Read the model definition and answer for the solid it produces. Units are mm, in the model's axes. Face numbers are marked on the shaded views. A direction names the side the tool comes from. Coordinates: 2 decimals unless noted, no trailing zeros. Order: outer loops, then holes, each group sorted by start corner. A loop starts at its lowest first (then second) coordinate and runs counter-clockwise, first axis right, second up. Notation, with made-up numbers: (-1.5, -17.5) -> (35.5, -17.5) arc R30 cw to (35.5, 17.5) -> close; hole circle Ø4 at (-36, 13). An arc over 180 degrees is marked (long way). Use CSV: the item, a comma, the result in double quotes.
```python
from build123d import *

# Parameters (mm, degrees)
EXTRUDE_1_DEPTH     = 14
SKETCH_3_W          = 34.989164417
SKETCH_3_H          = 23.7
EXTRUDE_2_DEPTH     = 1.99
SKETCH_4_W          = 19.73952378
SKETCH_4_H          = 14
CUT_EXTRUDE_1_DEPTH = 1.99
EXTRUDE_3_DEPTH     = 4.99
EXTRUDE_4_DEPTH     = 5.55
EXTRUDE_5_DEPTH     = 1.02
SKETCH_13_W         = 35
SKETCH_13_H         = 14
EXTRUDE_6_DEPTH     = 4
EXTRUDE_8_DEPTH     = 21
SKETCH_15_W         = 5
SKETCH_15_H         = 5.74
SKETCH_15_H_2       = 4
EXTRUDE_9_DEPTH     = 14
EXTRUDE_10_DEPTH    = 1
SKETCH_17_W         = 35
SKETCH_17_H         = 19
EXTRUDE_11_DEPTH    = 3
SKETCH_18_W         = 35
SKETCH_18_H         = 5
EXTRUDE_12_DEPTH    = 1
EXTRUDE_16_DEPTH    = 3
SKETCH_20_W         = 5.25
SKETCH_20_H         = 3.26
SKETCH_20_H_2       = 3
EXTRUDE_18_DEPTH    = 35
SKETCH_21_W         = 14
SKETCH_21_H         = 3.74
SKETCH_21_H_2       = 3.75
EXTRUDE_19_DEPTH    = 5
EXTRUDE_20_DEPTH    = 11
SKETCH_26_W         = 0.25
SKETCH_26_H         = 8.5
EXTRUDE_21_DEPTH    = 3
SKETCH_27_W         = 21
SKETCH_27_H         = 8.5
EXTRUDE_22_DEPTH    = 80
SKETCH_28_R         = 25
SKETCH_28_R_2       = 6
SKETCH_28_R_3       = 1.5
EXTRUDE_23_DEPTH    = 3


with BuildPart() as part:
    # 草图2 → 凸台-拉伸1 (new body)
    with BuildSketch(Plane.XY.offset(6)):
        Polygon((58.617261146, 15.562420382), (53.219585402, 15.562420382), (53.219585402, 12.262420382), (57.419585402, 12.262420382), (57.419585402, 8.862420382), (53.219585402, 8.862420382), (53.219585402, -6.137579618), (29.014936891, -6.137579618), (29.014936891, 8.862420382), (24.814936891, 8.862420382), (24.814936891, 12.262420382), (29.014936891, 12.262420382), (29.014936891, 15.562420382), (23.617261146, 15.562420382), (23.617261146, -8.137579618), (58.617261146, -8.137579618), align=None)
    extrude(amount=-EXTRUDE_1_DEPTH)

    # 草图3 → 凸台-拉伸2 (add)
    with BuildSketch(Plane(origin=(0, 0, -8), x_dir=(-1, 0, 0), z_dir=(0, 0, -1))):
        with Locations((-41.122678938, 3.712420382)):
            Rectangle(SKETCH_3_W, SKETCH_3_H)
    extrude(amount=-EXTRUDE_2_DEPTH)

    # 草图4 → 切除-拉伸1 (cut)
    with BuildSketch(Plane.XZ.offset(8.137579618)):
        with Locations((41.002259963, -1)):
            Rectangle(SKETCH_4_W, SKETCH_4_H)
    extrude(amount=-CUT_EXTRUDE_1_DEPTH, mode=Mode.SUBTRACT)

    # 草图7 → 凸台-拉伸3 (add)
    with BuildSketch(Plane(origin=(0, 15.562420382, 0), x_dir=(1, 0, 0), z_dir=(0, 1, 0))):
        Polygon((29.014936891, -6), (23.617261146, -6), (23.617261146, 8), (58.617261146, 8), (58.617261146, -6), (53.219585402, -6), (53.219585402, 6.01), (29.014936891, 6.01), align=None)
    extrude(amount=EXTRUDE_3_DEPTH)

    # 草图8 → 凸台-拉伸4 (add)
    with BuildSketch(Plane(origin=(0, 20.552420382, 0), x_dir=(1, 0, 0), z_dir=(0, 1, 0))):
        Polygon((23.617261146, -6), (29.014936891, -6), (29.014936891, 6.01), (44.953536614, 6.01), (44.953536614, -6), (58.617261146, -6), (58.617261146, 8), (23.617261146, 8), align=None)
    extrude(amount=EXTRUDE_4_DEPTH)

    # 草图11 → 凸台-拉伸5 (add)
    with BuildSketch(Plane(origin=(0, 26.102420382, 0), x_dir=(1, 0, 0), z_dir=(0, 1, 0))):
        with BuildLine():
            Line((51.35010895, 8), (58.617261146, 8))
            Line((58.617261146, 8), (58.617261146, -6))
            Line((58.617261146, -6), (52.21613159, -6))
            ThreePointArc((52.21613159, -6), (53.233588834, 1.089724187), (51.35010895, 8))
        make_face()
    extrude(amount=EXTRUDE_5_DEPTH)

    # 草图13 → 凸台-拉伸6 (add)
    with BuildSketch(Plane(origin=(0, 27.122420382, 0), x_dir=(1, 0, 0), z_dir=(0, 1, 0))):
        with Locations((41.117261146, 1)):
            Rectangle(SKETCH_13_W, SKETCH_13_H)
    extrude(amount=EXTRUDE_6_DEPTH)

    # 草图14 → 凸台-拉伸8 (add)
    with BuildSketch(Plane.ZY.offset(-23.617261146)):
        with BuildLine():
            Line((-8.78071096, 27.122420382), (-8, 27.122420382))
            Line((-8, 27.122420382), (-8, 31.122420382))
            Line((-8, 31.122420382), (-13, 31.122420382))
            Line((-13, 31.122420382), (-13, 30.862420382))
            ThreePointArc((-13, 30.862420382), (-10.180868928, 29.792829161), (-8.78071096, 27.122420382))
        make_face()
        with BuildLine():
            Line((-8, 26.102420382), (-8.78071096, 26.102420382))
            ThreePointArc((-8.78071096, 26.102420382), (-10.180868928, 23.432011603), (-13, 22.362420382))
            Line((-13, 22.362420382), (-13, 20.362420382))
            Line((-13, 20.362420382), (-8, 20.362420382))
            Line((-8, 20.362420382), (-8, 26.102420382))
        make_face()
    extrude(amount=-EXTRUDE_8_DEPTH)

    # 草图15 → 凸台-拉伸9 (add)
    with BuildSketch(Plane(origin=(44.617261146, 0, 0), x_dir=(0, 0, -1), z_dir=(1, 0, 0))):
        with Locations((10.5, 23.232420382)):
            Rectangle(SKETCH_15_W, SKETCH_15_H)
        with Locations((10.5, 29.122420382)):
            Rectangle(SKETCH_15_W, SKETCH_15_H_2)
    extrude(amount=EXTRUDE_9_DEPTH)

    # 草图16 → 凸台-拉伸10 (add)
    with BuildSketch(Plane(origin=(0, 26.102420382, 0), x_dir=(1, 0, 0), z_dir=(0, 1, 0))):
        with BuildLine():
            Line((47.481493106, 13), (58.617261146, 13))
            Line((58.617261146, 13), (58.617261146, 8))
            Line((58.617261146, 8), (51.2939955, 8))
            ThreePointArc((51.2939955, 8), (49.612839247, 10.671635002), (47.481493106, 13))
        make_face()
    extrude(amount=EXTRUDE_10_DEPTH)

    # 草图17 → 凸台-拉伸11 (add)
    with BuildSketch(Plane(origin=(0, 31.122420382, 0), x_dir=(1, 0, 0), z_dir=(0, 1, 0))):
        with Locations((41.117261146, 3.5)):
            Rectangle(SKETCH_17_W, SKETCH_17_H)
    extrude(amount=EXTRUDE_11_DEPTH)

    # 草图18 → 凸台-拉伸12 (add)
    with BuildSketch(Plane.XZ.offset(-20.362420382)):
        with Locations((41.117261146, -10.5)):
            Rectangle(SKETCH_18_W, SKETCH_18_H)
    extrude(amount=EXTRUDE_12_DEPTH)

    # 草图19 → 凸台-拉伸16 (add)
    with BuildSketch(Plane.ZY.offset(-23.617261146)):
        with BuildLine():
            Line((-8, 19.362420382), (-8, -8.137579618))
            Line((-8, -8.137579618), (6, -8.137579618))
            Line((6, -8.137579618), (6, 26.102420382))
            Line((6, 26.102420382), (-8.78071096, 26.102420382))
            ThreePointArc((-8.78071096, 26.102420382), (-17.25, 26.612420382), (-8.78071096, 27.122420382))
            Line((-8.78071096, 27.122420382), (6, 27.122420382))
            Line((6, 27.122420382), (6, 34.122420382))
            Line((6, 34.122420382), (-18.25, 34.122420382))
            Line((-18.25, 34.122420382), (-18.25, 19.362420382))
            Line((-18.25, 19.362420382), (-8, 19.362420382))
        make_face()
    extrude(amount=EXTRUDE_16_DEPTH)

    # 草图20 → 凸台-拉伸18 (add)
    with BuildSketch(Plane(origin=(23.617261146, 0, 0), x_dir=(0, 0, -1), z_dir=(1, 0, 0))):
        with Locations((15.625, 32.492420382)):
            Rectangle(SKETCH_20_W, SKETCH_20_H)
        with Locations((15.625, 20.862420382)):
            Rectangle(SKETCH_20_W, SKETCH_20_H_2)
    extrude(amount=EXTRUDE_18_DEPTH)

    # 草图21 → 凸台-拉伸19 (add)
    with BuildSketch(Plane(origin=(0, 0, -13), x_dir=(-1, 0, 0), z_dir=(0, 0, -1))):
        with Locations((-51.617261146, 28.992420382)):
            Rectangle(SKETCH_21_W, SKETCH_21_H)
        with Locations((-51.617261146, 24.237420382)):
            Rectangle(SKETCH_21_W, SKETCH_21_H_2)
    extrude(amount=EXTRUDE_19_DEPTH)

    # 草图22 → 凸台-拉伸20 (add)
    with BuildSketch(Plane(origin=(58.617261146, 0, 0), x_dir=(0, 0, -1), z_dir=(1, 0, 0))):
        Polygon((18, 27.102420382), (13, 27.102420382), (13, 26.155844896), (18, 26.155844896), (18, 22.362420382), (18.25, 22.362420382), (18.25, 30.862420382), (18, 30.862420382), align=None)
    extrude(amount=-EXTRUDE_20_DEPTH)

    # 草图26 → 凸台-拉伸21 (add)
    with BuildSketch(Plane.ZY.offset(-47.617261146)):
        with Locations((-18.125, 26.612420382)):
            Rectangle(SKETCH_26_W, SKETCH_26_H)
    extrude(amount=EXTRUDE_21_DEPTH)

    # 草图27 → 凸台-拉伸22 (add)
    with BuildSketch(Plane(origin=(0, 0, -18.25), x_dir=(-1, 0, 0), z_dir=(0, 0, -1))):
        Polygon((-47.617261146, 34.122420382), (-47.617261146, 30.862420382), (-47.617261146, 19.362420382), (-20.617261146, 19.362420382), (-20.617261146, 34.122420382), align=None)
        with Locations((-34.117261146, 26.612420382)):
            Rectangle(SKETCH_27_W, SKETCH_27_H, mode=Mode.SUBTRACT)
    extrude(amount=EXTRUDE_22_DEPTH)

    # 草图28 → 凸台-拉伸23 (add)
    with BuildSketch(Plane.ZY.offset(-20.617261146)):
        with Locations((-13, 26.612420382)):
            Circle(SKETCH_28_R)
        with Locations((-13, 26.612420382)):
            Circle(SKETCH_28_R_2, mode=Mode.SUBTRACT)
        with Locations((-13, 4.102420382)):
            Circle(SKETCH_28_R_3, mode=Mode.SUBTRACT)
        with Locations((-32.494231839, 15.357420382)):
            Circle(SKETCH_28_R_3, mode=Mode.SUBTRACT)
        with Locations((-32.494231839, 37.867420382)):
            Circle(SKETCH_28_R_3, mode=Mode.SUBTRACT)
        with Locations((-13, 49.122420382)):
            Circle(SKETCH_28_R_3, mode=Mode.SUBTRACT)
        with Locations((6.494231839, 37.867420382)):
            Circle(SKETCH_28_R_3, mode=Mode.SUBTRACT)
        with Locations((6.494231839, 15.357420382)):
            Circle(SKETCH_28_R_3, mode=Mode.SUBTRACT)
    extrude(amount=EXTRUDE_23_DEPTH)


solid = part.part
```
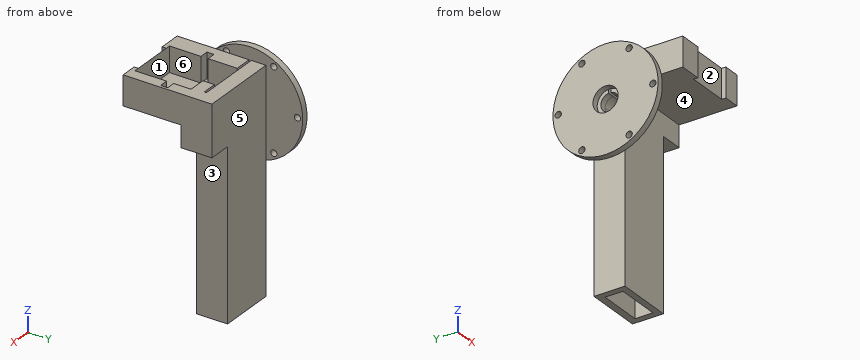
Item 1: The mould has two halves that part along Y. Classify the marked faces 1, 2 and 3: +Y half, -Y half, draft (parallel to the pull), parting line (faces both ways), or undercut.
Return value:
face 1,"undercut"
face 2,"-Y half"
face 3,"draft"
Item 2: A tool of negligible diameter and unlimited length cuts with its end or side. For the marked faces 4, 5 and 6, from which of +Z, -Z, +X, -X, +Y, -Y can it reach the whole face along a straight path? Write none if from no direction.
Return value:
face 4,"-Z, +X, -Y"
face 5,"+Z, -Z, +X, +Y"
face 6,"+Z"
Item 3: Find section C-C, the plane y = 46.5. Give the vertices of the cut face in (x, z).
Return value:
outline,"(17.62, -28.15) -> (20.62, -28.15) -> (20.62, 2.15) -> (17.62, 2.15) -> close"
Item 4: Each of these flat-tipped pins is pushed along its axis until it touches: P1, Ø4.5, axis at y = 30, z = -68.5, coming from the +X side; P2, Ø4, axis at y = 37.87, z = 6.49, coming from the +X side; P3, Ø9.5, axis at x = 38, z = -0.5, coming from the +Y side. Where does it stop, or does it pass through?
Return value:
P1,"stops at x = 47.62"
P2,"stops at x = 20.62"
P3,"stops at y = 34.12"
Item 5: Find section B-B, the plane z = -50. Give the vertices of the cut face in (x, y).
Return value:
outline,"(20.62, 19.36) -> (47.62, 19.36) -> (47.62, 34.12) -> (20.62, 34.12) -> close; hole (23.62, 22.36) -> (44.62, 22.36) -> (44.62, 30.86) -> (23.62, 30.86) -> close"
Item 6: Straight lines are drawn through the part: line 1 along Y through (x, z) = (18, -13); line 2 along Y through (x, z) = (36, -22); line 3 along X through (y, z) = (26, -55). For each, find the intervals that lie inside material, in ascending order.
Return value:
line 1,"y = 1.61 to 2.6, 5.6 to 20.61, 32.61 to 47.62, 50.62 to 51.61"
line 2,"y = 19.36 to 22.36, 30.86 to 34.12"
line 3,"x = 20.62 to 23.62, 44.62 to 47.62"
